Here's the drawing with two shaded views (mm, measured from the low corner). I have some questions. Round coordinates to 2 decimals unless told otherwise and drop trailing zeros. Write each loop counter-clockwise with the first axis right and the second up, starting at its lowest first coordinate (ties: lowest second). Pieces come first, ordered by that corner, then holes. Notation, with made-up numbers: (17.25, 86.25) - (38.25, 86.25) arc R31 ccw to (38.25, 123.25) - close; hole circle Ø4 at (44, 24). An arc over 180 degrees is marked (long way). Return JSON: item names as keys, results as strings. Group by question number.
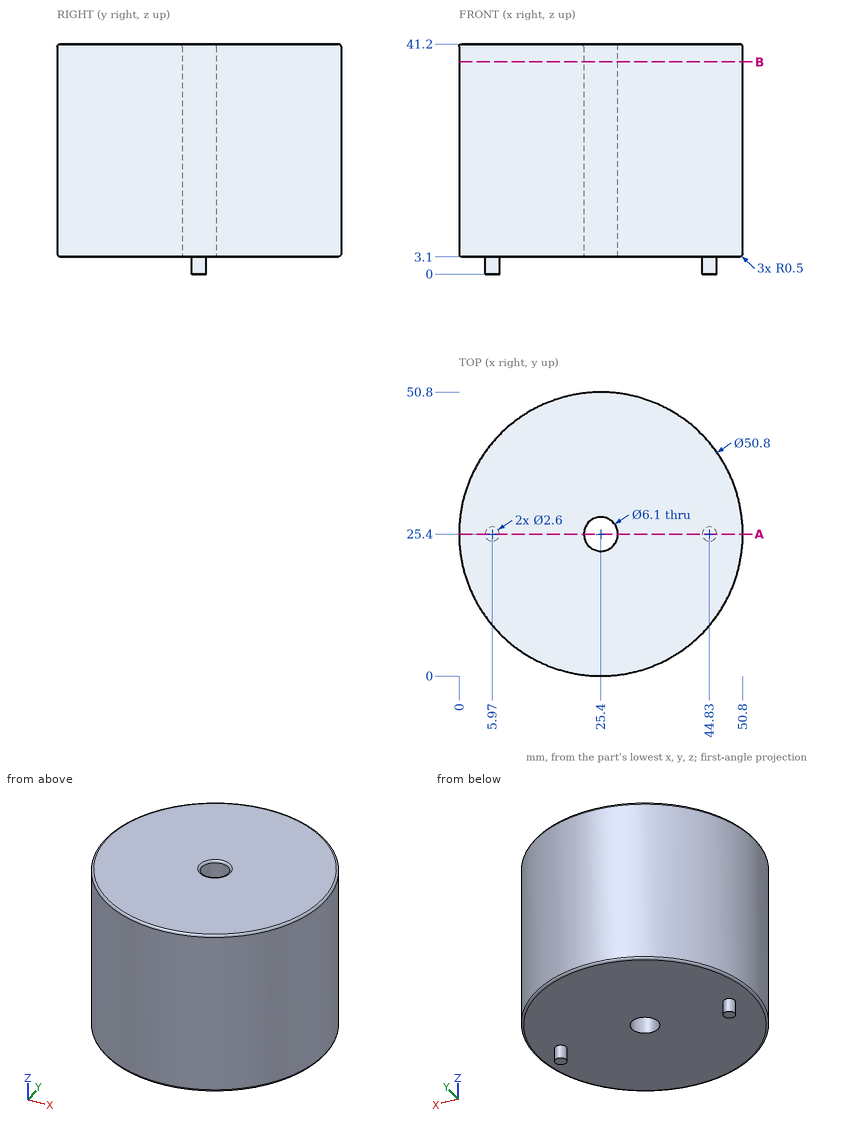
1) Will these pins go through, and if not, where does the flat tip stop? pin 1 Ø1 at (x, y) = (25.5, 21) entering from -Z; pin 2 Ø3 at (x, z) = (10.5, 36) entering from -Y; pin 3 Ø6 at (y, z) = (20, 29) entering from +X.
2) Imagine slicing it at B-B (z = 38). Please give me the cut outline in (x, y), plus the area to 3 significant figures.
3) I need wall thicknesses on line 1 along Y through (x, z) = (25.4, 12); line 2 along Z through (x, y) = (32, 15); line 3 along Y through (x, z) = (24, 11). Which ranges of each line are inside material? Lowest first, please.
4) Imagine slicing it at A-A (y = 25.4). Please give me the cut outline in (x, z).
Results found:
{
 "1": {"pin 1": "stops at z = 3.1", "pin 2": "stops at y = 3.82", "pin 3": "stops at x = 50.69"},
 "2": {"outline": "circle Ø50.8 at (25.4, 25.4); hole circle Ø6.1 at (25.4, 25.4)", "area": "2,000 mm²"},
 "3": {"line 1": "y = 0 to 22.35, 28.45 to 50.8", "line 2": "z = 3.1 to 41.2", "line 3": "y = 0.04 to 22.69, 28.11 to 50.76"},
 "4": {"outline": "(0, 3.6) arc R0.5 ccw to (0.5, 3.1) - (4.67, 3.1) - (4.67, 0) - (7.27, 0) - (7.27, 3.1) - (22.35, 3.1) - (22.35, 40.7) arc R0.5 ccw to (21.85, 41.2) - (0.5, 41.2) arc R0.5 ccw to (0, 40.7) - close; (28.45, 3.1) - (43.53, 3.1) - (43.53, 0) - (46.13, 0) - (46.13, 3.1) - (50.3, 3.1) arc R0.5 ccw to (50.8, 3.6) - (50.8, 40.7) arc R0.5 ccw to (50.3, 41.2) - (28.95, 41.2) arc R0.5 ccw to (28.45, 40.7) - close"}
}
